Check sheet for the modelled part. Datum: model origin and axes. Units: mm. A direction names the side the tool comes from. Round coordinates to 2 decimals unless told otherwise and drop trailing zeros. Write each loop counter-clockwise with the first axis right and the second up, starting at its lowest first coordinate (ties: lowest second). Pieces come first, ordered by that corner, then holes.
Item 1: Go/stop test with flat-tipped pins: pin 1 Ø6 at (x, z) = (-46.5, -18.5) entering from +Y; pin 2 Ø3.5 at (y, z) = (19, -38.5) entering from -X; pin 3 Ø1.5 at (x, z) = (7, 34) entering from +Y. Record where each tip stops, or that it passes through.
Item 2: Tool access check on faces 5 (the flat face through (-8, 25, 35)), 6 (the flat face through (-71, 25, -16)), 7 (the cylindrical face through (48.311, 26.829, 29.375)), 8 (the flat face through (-12, 50, -39)), 9 (the flat face through (-1, 1, -20)). Record the directions out of +Z, -Z, +X, -X, +Y, -Y that give a thin tool (end or side, any length) a straight path to the whole face; none if there is none.
Item 3: Cross-section at D-D on x = 15.5. Enter the section's corners in (y, z).
Item 4: Cross-section at C-C on y = 22. Enter the section's corners in (x, z), plus the area to 3 significant figures.
Item 5: Release check for a two-part mould opening along Z. For faces 1 (the flat face through (-75, 25, -26)), 2 (the flat face through (49, 1, 0)), 3 (the cylindrical face through (-65.93, 45.07, 30.5)), 4 (the flat face through (-71, 37, -21)) record: +Z half, -Z half, draft (parallel to the pull), parting line (faces both ways), or undercut.
Item 6: Cross-section at A-A on x = -20.5. Enter the section's corners in (y, z).
Item 7: Material ranges on line 1 (X direction, y = 11.5, z = 9.5); line 2 (X direction, y = 2.25, z = -27.5); line 3 (X direction, y = 22, z = -17), recorded low to high.
Item 8: Cross-section at B-B on z = -4. Enter the section's corners in (x, y).
from build123d import *

# Parameters (mm, degrees)
SKETCH_1_R          = 1.5
EXTRUDE_1_DEPTH     = 3
SKETCH_2_W          = 123
SKETCH_2_H          = 75
EXTRUDE_2_DEPTH     = 47
SKETCH_3_W          = 6.652297382
SKETCH_3_H          = 12.01949186
CUT_EXTRUDE_1_DEPTH = 20
EXTRUDE_3_DEPTH     = 47
SKETCH_5_R          = 1.5
CUT_EXTRUDE_2_DEPTH = 10
SKETCH_7_W          = 4
SKETCH_7_H          = 24
EXTRUDE_4_DEPTH     = 8
SKETCH_8_W          = 4
SKETCH_8_H          = 24
EXTRUDE_5_DEPTH     = 10
SKETCH_9_W          = 14
SKETCH_9_H          = 4
EXTRUDE_6_DEPTH     = 8
SKETCH_10_W         = 29.551054495
SKETCH_10_H         = 15
CUT_EXTRUDE_3_DEPTH = 10
SKETCH_11_W         = 18
SKETCH_11_H         = 14
CUT_EXTRUDE_4_DEPTH = 10


with BuildPart() as part:
    # Эскиз1 → Бобышка-Вытянуть1 (new body)
    with BuildSketch(Plane(origin=(0, 0, 0), x_dir=(1, 0, 0), z_dir=(0, 1, 0))):
        Polygon((54, -3.949274275), (54, 40), (-69, 40), (-69, -35), (54, -35), align=None)
        with Locations(Location((-46.5, 27.5, 0), (0, 0, 270))):
            Circle(SKETCH_1_R, mode=Mode.SUBTRACT)
        with Locations(Location((-46.5, -27.5, 0), (0, 0, 270))):
            Circle(SKETCH_1_R, mode=Mode.SUBTRACT)
        with Locations(Location((46.5, 27.5, 0), (0, 0, 270))):
            Circle(SKETCH_1_R, mode=Mode.SUBTRACT)
        with Locations(Location((46.5, -27.5, 0), (0, 0, 270))):
            Circle(SKETCH_1_R, mode=Mode.SUBTRACT)
        Polygon((-49, 20), (-49, -20), (0, -20), (49, -20), (49, 20), (0, 20), align=None, mode=Mode.SUBTRACT)
    extrude(amount=EXTRUDE_1_DEPTH)

    # Эскиз2 → Бобышка-Вытянуть2 (add)
    with BuildSketch(Plane(origin=(0, 3, 0), x_dir=(1, 0, 0), z_dir=(0, 1, 0))):
        with Locations((-7.5, 2.5)):
            Rectangle(SKETCH_2_W, SKETCH_2_H)
        Polygon((-50, -32), (51, -32), (51, 37), (-50, 37), (-50, 0), align=None, mode=Mode.SUBTRACT)
        Polygon((-66, 37), (-53, 37), (-53, 0), (-53, -32), (-66, -32), align=None, mode=Mode.SUBTRACT)
    extrude(amount=EXTRUDE_2_DEPTH)

    # Эскиз3 → Вырез-Вытянуть1 (cut)
    with BuildSketch(Plane(origin=(0, 50, 0), x_dir=(1, 0, 0), z_dir=(0, 1, 0))):
        with Locations((-51.818044752, 16.773138265)):
            Rectangle(SKETCH_3_W, SKETCH_3_H)
    extrude(amount=-CUT_EXTRUDE_1_DEPTH, mode=Mode.SUBTRACT)

    # Эскиз4 → Бобышка-Вытянуть3 (add)
    with BuildSketch(Plane(origin=(0, 50, 0), x_dir=(1, 0, 0), z_dir=(0, 1, 0))):
        with BuildLine():
            Line((-69, 32), (-69, 40))
            Line((-69, 40), (-61, 40))
            ThreePointArc((-61, 40), (-63.343145751, 34.343145751), (-69, 32))
        make_face()
        with BuildLine():
            Line((46, 40), (54, 40))
            Line((54, 40), (54, 32))
            ThreePointArc((54, 32), (48.343145751, 34.343145751), (46, 40))
        make_face()
        with BuildLine():
            Line((-69, -27), (-69, -35))
            Line((-69, -35), (-61, -35))
            ThreePointArc((-61, -35), (-63.343145751, -29.343145751), (-69, -27))
        make_face()
        with BuildLine():
            Line((54, -27), (54, -35))
            Line((54, -35), (46, -35))
            ThreePointArc((46, -35), (48.343145751, -29.343145751), (54, -27))
        make_face()
    extrude(amount=-EXTRUDE_3_DEPTH)

    # Эскиз5 → Вырез-Вытянуть2 (cut)
    with BuildSketch(Plane(origin=(0, 50, 0), x_dir=(1, 0, 0), z_dir=(0, 1, 0))):
        with Locations(Location((-66, 37, 0), (0, 0, 270))):
            Circle(SKETCH_5_R)
        with Locations(Location((-66, -32, 0), (0, 0, 270))):
            Circle(SKETCH_5_R)
        with Locations(Location((51, -32, 0), (0, 0, 270))):
            Circle(SKETCH_5_R)
        with Locations(Location((51, 37, 0), (0, 0, 270))):
            Circle(SKETCH_5_R)
    extrude(amount=-CUT_EXTRUDE_2_DEPTH, mode=Mode.SUBTRACT)

    # Эскиз7 → Бобышка-Вытянуть4 (add)
    with BuildSketch(Plane.ZY.offset(69)):
        with Locations((-14, 25)):
            Rectangle(SKETCH_7_W, SKETCH_7_H)
    extrude(amount=EXTRUDE_4_DEPTH)

    # Эскиз8 → Бобышка-Вытянуть5 (add)
    with BuildSketch(Plane(origin=(0, 0, -16), x_dir=(-1, 0, 0), z_dir=(0, 0, -1))):
        with Locations((75, 25)):
            Rectangle(SKETCH_8_W, SKETCH_8_H)
    extrude(amount=EXTRUDE_5_DEPTH)

    # Эскиз9 → Бобышка-Вытянуть6 (add)
    with BuildSketch(Plane.ZY.offset(69)):
        with Locations((-19, 39)):
            Rectangle(SKETCH_9_W, SKETCH_9_H)
        with Locations((-19, 11)):
            Rectangle(SKETCH_9_W, SKETCH_9_H)
    extrude(amount=EXTRUDE_6_DEPTH)

    # Эскиз10 → Вырез-Вытянуть3 (cut)
    with BuildSketch(Plane.XY.offset(35)):
        with Locations((10.188847336, 42.5)):
            Rectangle(SKETCH_10_W, SKETCH_10_H)
    extrude(amount=-CUT_EXTRUDE_3_DEPTH, mode=Mode.SUBTRACT)

    # Эскиз11 → Вырез-Вытянуть4 (cut)
    with BuildSketch(Plane(origin=(0, 0, -40), x_dir=(-1, 0, 0), z_dir=(0, 0, -1))):
        with Locations((21.719997663, 22.286107602)):
            Rectangle(SKETCH_11_W, SKETCH_11_H)
    extrude(amount=-CUT_EXTRUDE_4_DEPTH, mode=Mode.SUBTRACT)


solid = part.part
Response values:
1. pin 1: stops at y = 3
1. pin 2: stops at x = -69
1. pin 3: stops at y = 35
2. face 5: +Z, +X, -X, +Y, -Y
2. face 6: -Z
2. face 7: +Y
2. face 8: +Z, -Z, +X, -X, +Y
2. face 9: +Y, -Y
3. outline: (0, -40) - (50, -40) - (50, -37) - (3, -37) - (3, -20) - (0, -20) - close; (0, 20) - (3, 20) - (3, 32) - (35, 32) - (35, 35) - (0, 35) - close
4. outline: (-77, -26) - (-73, -26) - (-73, -16) - (-69, -16) - (-69, -40) - (-30.72, -40) - (-30.72, -37) - (-50, -37) - (-50, 32) - (46.58, 32) arc R8 ccw to (51, 27.58) - (51, -32.58) arc R8 ccw to (46.58, -37) - (-12.72, -37) - (-12.72, -40) - (54, -40) - (54, 35) - (-69, 35) - (-69, -12) - (-77, -12) - close; hole (-66, -32.58) arc R8 cw to (-61.58, -37) - (-53, -37) - (-53, 32) - (-61.58, 32) arc R8 cw to (-66, 27.58) - close
4. area: 1,430 mm2
5. face 1: -Z half
5. face 2: undercut
5. face 3: undercut
5. face 4: draft
6. outline: (0, -40) - (15.29, -40) - (15.29, -37) - (3, -37) - (3, -20) - (0, -20) - close; (0, 20) - (3, 20) - (3, 32) - (50, 32) - (50, 35) - (0, 35) - close; (29.29, -40) - (50, -40) - (50, -37) - (29.29, -37) - close
7. line 1: x = -69 to -66, -53 to -50, 51 to 54
7. line 2: x = -69 to -48, -45 to 45, 48 to 54
7. line 3: x = -77 to -73, -69 to -66, -53 to -50, 51 to 54
8. outline: (-69, 0) - (-49, 0) - (-49, 3) - (-50, 3) - (-50, 50) - (-53, 50) - (-53, 3) - (-66, 3) - (-66, 50) - (-69, 50) - close; (49, 0) - (54, 0) - (54, 50) - (51, 50) - (51, 3) - (49, 3) - close
